Can you work these out from the model? Positions are in its coordinate system, mm. Face numbers are marked on the shaded views. A direction names the side the tool comes from. Give positions to 0.01 mm unless a question says otherwise; leave off trailing zeros. Write each loop counter-clockwise with the first axis right and the second up, starting at its lowest first coordinate (ties: lowest second). Pieces come first, ordered by that corner, then holes. Notation, with made-up numbers: M -1.5,-23.75 L 23.5,-23.75 A24 cw 23.5,6.25 Z; hole C -33.75,-38 d5. An arc over 180 degrees is marked long. Answer as CSV lines item,"result". Start each with the question number.
```python
from build123d import *

# Parameters (mm, degrees)
EXTRUDE_1_DEPTH     = 3.7
CUT_EXTRUDE_1_REACH = 37.162
SKETCH_2_W          = 4.6
SKETCH_2_H          = 7.4
SKETCH_3_W          = 25.755
SKETCH_3_H          = 2
EXTRUDE_2_DEPTH     = 1
SKETCH_4_W          = 6.255
SKETCH_4_H          = 7.9
SKETCH_4_W_2        = 2.95
EXTRUDE_3_DEPTH     = 10.4
SKETCH_5_W          = 1.725
SKETCH_5_H          = 7.9
EXTRUDE_4_DEPTH     = 3
CUT_EXTRUDE_START   = -7.9
SKETCH_9_W          = 2.95
SKETCH_9_H          = 9.4
CUT_EXTRUDE_4_DEPTH = 7.9
FILLET_2_R          = 0.4
CUT_EXTRUDE_5_DEPTH = 7.9
CUT_EXTRUDE_START_2 = -25.755
SKETCH_12_W         = 1
SKETCH_12_H         = 2
CUT_EXTRUDE_6_DEPTH = 25.755
EXTRUDE_START       = -3.7
SKETCH_13_W         = 25.755
SKETCH_13_H         = 1.055
EXTRUDE_6_DEPTH     = 3.7
CUT_REVOLVE_1_ANGLE = 180
SKETCH_16_W         = 25.755
SKETCH_16_H         = 3.055
EXTRUDE_7_DEPTH     = 0.5


with BuildPart() as part:
    # ｽｹｯﾁ1 → ﾎﾞｽ - 押し出し1 (new body)
    with BuildSketch(Plane.XY):
        Polygon((0, 0), (12.75, 0), (25.755, 0), (25.755, 23.65), (12.75, 23.65), (0, 23.65), align=None)
    extrude(amount=EXTRUDE_1_DEPTH)

    # ｽｹｯﾁ2 → ｶｯﾄ - 押し出し1 (cut, up to next)
    with BuildSketch(Plane.XY.offset(3.7), mode=Mode.PRIVATE) as cut_extrude_1_sk1:
        with Locations((6.38, 11.825)):
            Rectangle(SKETCH_2_W, SKETCH_2_H)
    cut_extrude_1_tool1 = extrude(cut_extrude_1_sk1.sketch, amount=-CUT_EXTRUDE_1_REACH, mode=Mode.PRIVATE) & part.part
    # ｽｹｯﾁ2 → ｶｯﾄ - 押し出し1 (cut, up to next)
    with BuildSketch(Plane.XY.offset(3.7), mode=Mode.PRIVATE) as cut_extrude_1_sk2:
        with Locations((19.375, 11.825)):
            Rectangle(SKETCH_2_W, SKETCH_2_H)
    cut_extrude_1_tool2 = extrude(cut_extrude_1_sk2.sketch, amount=-CUT_EXTRUDE_1_REACH, mode=Mode.PRIVATE) & part.part
    add(cut_extrude_1_tool1.solids().sort_by_distance((6.38, 11.825, 3.7))[0], mode=Mode.SUBTRACT)
    add(cut_extrude_1_tool2.solids().sort_by_distance((19.375, 11.825, 3.7))[0], mode=Mode.SUBTRACT)

    # ｽｹｯﾁ3 → ﾎﾞｽ - 押し出し2 (add)
    with BuildSketch(Plane.XY.offset(3.7)):
        with Locations((12.8775, 22.65)):
            Rectangle(SKETCH_3_W, SKETCH_3_H)
        with Locations((12.8775, 1)):
            Rectangle(SKETCH_3_W, SKETCH_3_H)
    extrude(amount=EXTRUDE_2_DEPTH)

    # ｽｹｯﾁ4 → ﾎﾞｽ - 押し出し3 (add)
    with BuildSketch(Plane.XY.offset(3.7)):
        with Locations((12.8775, 11.825)):
            Rectangle(SKETCH_4_W, SKETCH_4_H)
        with Locations((1.475, 11.825)):
            Rectangle(SKETCH_4_W_2, SKETCH_4_H)
        with Locations((24.28, 11.825)):
            Rectangle(SKETCH_4_W_2, SKETCH_4_H)
    extrude(amount=EXTRUDE_3_DEPTH)

    # ｽｹｯﾁ5 → ﾎﾞｽ - 押し出し4 (add)
    with BuildSketch(Plane.XY.offset(14.1)):
        with Locations((16.8675, 11.825)):
            Rectangle(SKETCH_5_W, SKETCH_5_H)
        with Locations((8.8875, 11.825)):
            Rectangle(SKETCH_5_W, SKETCH_5_H)
    extrude(amount=-EXTRUDE_4_DEPTH)

    # ｽｹｯﾁ9 → ｶｯﾄ - 押し出し4 (cut)
    with BuildSketch(Plane.XZ.offset(-7.875).offset(CUT_EXTRUDE_START)):
        with Locations((1.475, 9.4)):
            Rectangle(SKETCH_9_W, SKETCH_9_H)
        with Locations((24.28, 9.4)):
            Rectangle(SKETCH_9_W, SKETCH_9_H)
    extrude(amount=CUT_EXTRUDE_4_DEPTH, mode=Mode.SUBTRACT)

    # ﾌｨﾚｯﾄ2
    fillet_2_edges = [part.edges().sort_by_distance(p)[0] for p in [
        (2.95, 11.825, 4.7),
        (22.805, 11.825, 4.7),
    ]]
    fillet(fillet_2_edges, radius=FILLET_2_R)

    # ｽｹｯﾁ11 → ｶｯﾄ - 押し出し5 (cut)
    with BuildSketch(Plane.XZ.offset(-7.875).offset(CUT_EXTRUDE_START)):
        with BuildLine():
            Line((2.95, 3.7), (2.95, 4.3))
            ThreePointArc((2.95, 4.3), (2.832842712, 4.582842712), (2.55, 4.7))
            Line((2.55, 4.7), (0, 4.7))
            Line((0, 4.7), (0, 3.7))
            Line((0, 3.7), (2.95, 3.7))
        make_face()
        with BuildLine():
            Line((25.755, 4.7), (23.205, 4.7))
            ThreePointArc((23.205, 4.7), (22.922157288, 4.582842712), (22.805, 4.3))
            Line((22.805, 4.3), (22.805, 3.7))
            Line((22.805, 3.7), (25.755, 3.7))
            Line((25.755, 3.7), (25.755, 4.7))
        make_face()
    extrude(amount=CUT_EXTRUDE_5_DEPTH, mode=Mode.SUBTRACT)

    # ｽｹｯﾁ12 → ｶｯﾄ - 押し出し6 (cut)
    with BuildSketch(Plane.ZY.offset(CUT_EXTRUDE_START_2)):
        with Locations((4.2, 22.65)):
            Rectangle(SKETCH_12_W, SKETCH_12_H)
        with Locations((4.2, 1)):
            Rectangle(SKETCH_12_W, SKETCH_12_H)
    extrude(amount=CUT_EXTRUDE_6_DEPTH, mode=Mode.SUBTRACT)

    # ｽｹｯﾁ13 → ﾎﾞｽ - 押し出し6 (add)
    with BuildSketch(Plane(origin=(0, 0, 0), x_dir=(-1, 0, 0), z_dir=(0, 0, -1)).offset(EXTRUDE_START)):
        with Locations((-12.8775, 24.1775)):
            Rectangle(SKETCH_13_W, SKETCH_13_H)
        with Locations((-12.8775, -0.5275)):
            Rectangle(SKETCH_13_W, SKETCH_13_H)
    extrude(amount=EXTRUDE_6_DEPTH)

    # ｽｹｯﾁ14 → ｶｯﾄ - 回転1 (revolve, cut)
    with BuildSketch(Plane(origin=(25.755, 0, 0), x_dir=(0, 0, -1), z_dir=(1, 0, 0))):
        with BuildLine():
            Line((-1.85, 21.255), (-1.85, 19.555))
            ThreePointArc((-1.85, 19.555), (-2.7, 20.405), (-1.85, 21.255))
        make_face()
        with BuildLine():
            Line((-1.85, 2.395), (-1.85, 4.095))
            ThreePointArc((-1.85, 4.095), (-2.7, 3.245), (-1.85, 2.395))
        make_face()
    cut_revolve_1 = revolve(axis=Axis((25.755, 21.255, 1.85), (0, -1, 0)), revolution_arc=CUT_REVOLVE_1_ANGLE, mode=Mode.SUBTRACT)

    # ﾐﾗｰ1: ｶｯﾄ - 回転1 across plane
    add(cut_revolve_1.mirror(Plane(origin=(12.8775, 0, 0), x_dir=(0, 0, 1), z_dir=(1, 0, 0))), mode=Mode.SUBTRACT)

    # ｽｹｯﾁ15 → ｶｯﾄ - 回転2 (revolve, cut)
    with BuildSketch(Plane(origin=(0, 24.705, 0), x_dir=(1, 0, 0), z_dir=(0, 1, 0))):
        with BuildLine():
            Line((3.4475, -1.85), (5.1475, -1.85))
            ThreePointArc((5.1475, -1.85), (4.2975, -2.7), (3.4475, -1.85))
        make_face()
        with BuildLine():
            Line((22.3075, -1.85), (20.6075, -1.85))
            ThreePointArc((20.6075, -1.85), (21.4575, -2.7), (22.3075, -1.85))
        make_face()
    cut_revolve_2 = revolve(axis=Axis((3.4475, 24.705, 1.85), (1, 0, 0)), mode=Mode.SUBTRACT)

    # ﾐﾗｰ2: ｶｯﾄ - 回転2 across plane
    add(cut_revolve_2.mirror(Plane(origin=(0, 11.825, 0), x_dir=(0, 0, 1), z_dir=(0, -1, 0))), mode=Mode.SUBTRACT)

    # ｽｹｯﾁ16 → ﾎﾞｽ - 押し出し7 (add)
    with BuildSketch(Plane.XY.offset(3.7)):
        with Locations((12.8775, 23.1775)):
            Rectangle(SKETCH_16_W, SKETCH_16_H)
        with Locations((12.8775, 0.4725)):
            Rectangle(SKETCH_16_W, SKETCH_16_H)
    extrude(amount=EXTRUDE_7_DEPTH)


solid = part.part
```
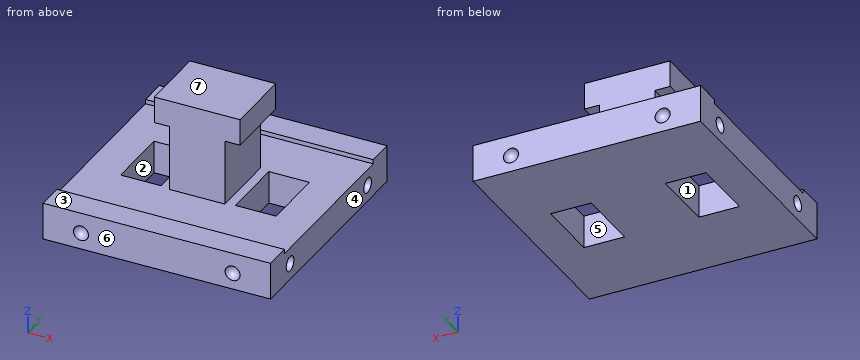
1) I want a section at D-D, the plane y = 18. Please give me the cut outline in (x, z) (3 decimals).
2) I want a section at A-A, the plane y = 10.75. Please give me the cut outline in (x, z) (3 decimals).
3) On a 3-axis mill with a long thin cutter (end or side, diameter ignored), from which of +Z, -Z, +X, -X, +Y, -Y can I reach the whole of each face in a straight line? I mean the marked faces 1, 2, 3 and 4. Say none if no direction works.
4) I want a section at B-B, the plane x = 15. Please give me the cut outline in (y, z) (3 decimals), then the cut area to 3 significant figures.
5) I'm going to push flat-ended pins straight in: P1, Ø6, axis at y = 14, z = 6, coming from the +X side (3 decimals); P2, Ø1, axis at x = 17.5, y = 19, coming from the +Z side; P3, Ø4, axis at x = 15, z = 8, coming from the +Y side (3 decimals); P4, Ø3.5, axis at x = 15.5, y = 0, coming from the +Z side. Where does each tip first touch, or does it pass through?
6) I want a section at C-C, the plane z = 9. Please give me the cut outline in (x, y) (3 decimals).
7) Thinking about a two-plate mould opening in Y: for the marked faces 5, 6 and 7, which applies, released by +Y, released by -Y, zero draft, split by the parting line, or undercut?
8) I need wall thicknesses on L1, parallel to Y at x = 20.5, z = 3.75 (3 decimals); L2, parallel to Y at x = 10.25, z = 12.5 (3 decimals); L3, parallel to Z at x = 7.5, y = 21.5. Which ranges of each line are inside material? Lowest first, please. Write a range as from..to.
Values found:
1,outline,"M 0,0 L 25.755,0 L 25.755,3.7 L 0,3.7 Z"
2,outline,"M 0,0 L 4.08,0 L 4.08,3.7 L 0,3.7 Z; M 8.025,11.1 L 9.75,11.1 L 9.75,3.7 L 8.68,3.7 L 8.68,0 L 17.075,0 L 17.075,3.7 L 16.005,3.7 L 16.005,11.1 L 17.73,11.1 L 17.73,14.1 L 8.025,14.1 Z; M 21.675,0 L 25.755,0 L 25.755,3.7 L 21.675,3.7 Z"
3,face 1,"-Z"
3,face 2,"+Z, -Z"
3,face 3,"+Z, +X, -X, -Y"
3,face 4,"+Z, -Z, +X, +Y, -Y"
4,outline,"M -1.055,0 L 24.705,0 L 24.705,4.2 L 21.65,4.2 L 21.65,3.7 L 15.775,3.7 L 15.775,14.1 L 7.875,14.1 L 7.875,3.7 L 2,3.7 L 2,4.2 L -1.055,4.2 Z"
4,area,"181 mm²"
5,P1,"stops at x = 25.755"
5,P2,"stops at z = 3.7"
5,P3,"stops at y = 15.775"
5,P4,"stops at z = 4.2"
6,outline,"M 9.75,7.875 L 16.005,7.875 L 16.005,15.775 L 9.75,15.775 Z"
7,face 5,"undercut"
7,face 6,"released by -Y"
7,face 7,"zero draft"
8,L1,"y = -1.055..2, 21.65..24.705"
8,L2,"y = 7.875..15.775"
8,L3,"z = 0..3.7"
